For this review, take the finished solid that the model builds, in its own axes (mm). A direction names the side the tool comes from. Coordinates: 2 decimals unless noted, no trailing zeros. Loops run counter-clockwise (first coordinate to the right, second up) from the corner with the lowest first, then second, coordinate; pieces in that order, holes last. Notation, with made-up numbers: M -35.75,-31.5 L -0.75,-31.5 A19 ccw -0.75,-20.5 Z; hole C 20,13.25 d8. An arc over 180 degrees is marked long. Answer as a JSON object with one key per item and string values. Group by question number.
Item 1: Wall thickness on L1, parallel to Y at x = 0.25, z = -3.75; L2, parallel to X at y = -3.5, z = 2.75; L3, parallel to Z at x = -8.5, y = 2.5: over which ranges is each line inside the solid? List them lowest first. Write a range as from..to.
Item 2: Add section B-B (x = -7.25). State the section outline as (y, z) points.
Item 3: Insertion check: pin 1 (5 mm diameter, centred on y = -5, z = -2, fed in from -X); pin 2 (5 mm diameter, centred on y = 4.5, z = -6, fed in from +X); pin 3 (1 mm diameter, centred on y = -2, z = -5, fed in from +X); pin 4 (3.5 mm diameter, centred on x = -7.72, y = -4.07, fed in from -Z). Each pin has a flat end and moves straight along its axis. Give the tip position at first contact, or say it passes through.
Item 4: Tool access review of faces 1 (the face through (1.4, -6.32, -4.93)), 2 (the face through (0, -6.5, 1)): name each direction out of +Z, -Z, +X, -X, +Y, -Y from which nothing blocks a thin tool from reaching the whole face with its end or side.
Item 5: Mouldability with a two-part tool opening along X and no side actions: class faces 3 (the face through (-9.93, 5.9, 1.52)), 4 (the face through (-4.83, 1.52, -5.07)), 5 (the face through (9.93, 5.9, 1.52)) as +X half, -X half, draft (parallel to the pull), parting line (faces both ways), or undercut.
Item 6: Add section C-C (z = 0.25). State the section outline as (x, y) points (3 decimals).
Item 7: Add section A-A (y = 0). State the section outline as (x, z) points (3 decimals).
Item 8: Add section D-D (x = 0). State the section outline as (y, z) points (3 decimals), then the cut area to 3 significant figures.
from build123d import *

# Parameters (mm, degrees)
ESQUISSE1_W             = 21
ESQUISSE1_H             = 13
BOSS_EXTRU_1_DEPTH      = 3
CONG_1_R                = 2
ESQUISSE2_R             = 1.555
ENL_V_MAT_EXTRU_1_DEPTH = 4
ESQUISSE3_R             = 6.475
BOSS_EXTRU_2_DEPTH      = 10
ESQUISSE4_R             = 5.065
ENL_V_MAT_EXTRU_2_DEPTH = 10


with BuildPart() as part:
    # Esquisse1 → Boss.-Extru.1 (new body)
    with BuildSketch(Plane.XY):
        Rectangle(ESQUISSE1_W, ESQUISSE1_H)
    extrude(amount=BOSS_EXTRU_1_DEPTH)

    # Congé1
    cong_1_edges = [part.edges().sort_by_distance(p)[0] for p in [
        (-10.5, 6.5, 1.5),
        (10.5, 6.5, 1.5),
        (10.5, -6.5, 1.5),
        (-10.5, -6.5, 1.5),
    ]]
    fillet(cong_1_edges, radius=CONG_1_R)

    # Esquisse2 → Enlèv. mat.-Extru.1 (cut, through all)
    with BuildSketch(Plane.XY.offset(3)):
        with Locations((-7.725, -4.074069474)):
            Circle(ESQUISSE2_R)
        with Locations((7.835, -4.074069474)):
            Circle(ESQUISSE2_R)
    extrude(amount=-ENL_V_MAT_EXTRU_1_DEPTH, mode=Mode.SUBTRACT)

    # Esquisse3 → Boss.-Extru.2 (add)
    with BuildSketch(Plane(origin=(0, 0, 0), x_dir=(-1, 0, 0), z_dir=(0, 0, -1))):
        Circle(ESQUISSE3_R)
    extrude(amount=BOSS_EXTRU_2_DEPTH)

    # Esquisse4 → Enlèv. mat.-Extru.2 (cut)
    with BuildSketch(Plane(origin=(0, 0, -10), x_dir=(-1, 0, 0), z_dir=(0, 0, -1))):
        Circle(ESQUISSE4_R)
    extrude(amount=-ENL_V_MAT_EXTRU_2_DEPTH, mode=Mode.SUBTRACT)


solid = part.part
From the geometry:
{
 "1": {"L1": "y = -6.47..-5.06, 5.06..6.47", "L2": "x = -10.5..-9.17, -6.28..6.39, 9.28..10.5", "L3": "z = 0..3"},
 "2": {"outline": "M -6.5,0 L -5.55,0 L -5.55,3 L -6.5,3 Z; M -2.59,0 L 6.5,0 L 6.5,3 L -2.59,3 Z"},
 "3": {"pin 1": "stops at x = -10.5", "pin 2": "stops at x = 6.16", "pin 3": "stops at x = 6.3", "pin 4": "stops at z = 0"},
 "4": {"face 1": "-Z", "face 2": "+Z, -Z, +X, -X, -Y"},
 "5": {"face 3": "-X half", "face 4": "undercut", "face 5": "+X half"},
 "6": {"outline": "M -10.5,-4.5 A2 ccw -8.5,-6.5 L 8.5,-6.5 A2 ccw 10.5,-4.5 L 10.5,4.5 A2 ccw 8.5,6.5 L -8.5,6.5 A2 ccw -10.5,4.5 Z; hole C -7.725,-4.074 d3.11; hole C 7.835,-4.074 d3.11"},
 "7": {"outline": "M -10.5,0 L -6.475,0 L -6.475,-10 L -5.065,-10 L -5.065,0 L 5.065,0 L 5.065,-10 L 6.475,-10 L 6.475,0 L 10.5,0 L 10.5,3 L -10.5,3 Z"},
 "8": {"outline": "M -6.5,0 L -6.475,0 L -6.475,-10 L -5.065,-10 L -5.065,0 L 5.065,0 L 5.065,-10 L 6.475,-10 L 6.475,0 L 6.5,0 L 6.5,3 L -6.5,3 Z", "area": "67.2 mm²"}
}
